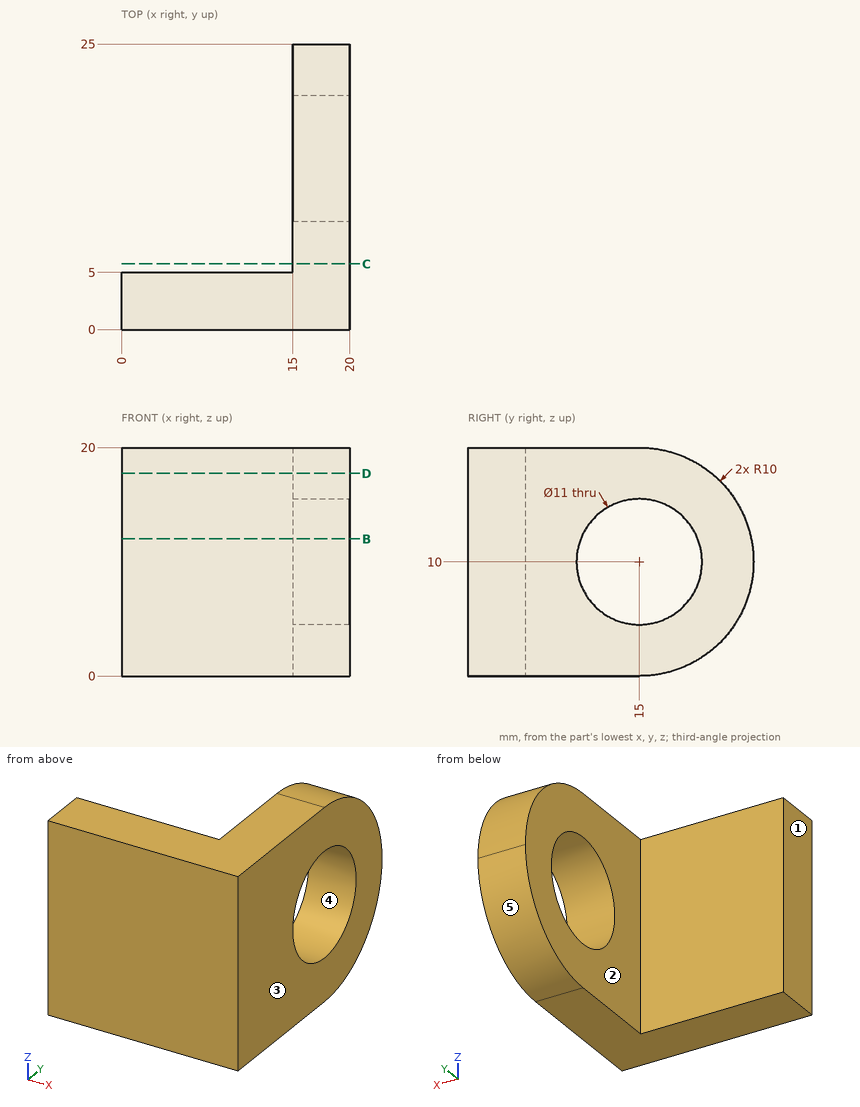
Geometry: see drawing. Coordinates: mm, zero at the bounding-box minimum. A direction names the side the tool comes from. Coordinates: 2 decimals unless noted, no trailing zeros. Order: outer loops, then holes, each group sorted by start corner. A loop starts at its lowest first (then second) coordinate and runs counter-clockwise, first axis right, second up. Notation, with made-up numbers: (89, 47.5) - (130, 47.5) arc R10 ccw to (130, 53.5) - close; hole circle Ø2 at (30.25, 41.25). An arc over 180 degrees is marked (long way). Return JSON: item names as keys, results as strings.
Q1. Access query for the marked faces 1 and 2. Directions: +Z, -Z, +X, -X, +Y, -Y. A direction counts if a zero-diameter tool reaches every point of the face in a straight line with its end or side. Return the directions, or none.
The answers:
{"face 1": "+Z, -Z, -X, +Y, -Y", "face 2": "+Z, -Z, -X, +Y"}
Q2. Cut plane C-C (y = 5.75). Return loops of the section in (x, z), then the cut area to 3 significant figures.
The answers:
{"outline": "(15, 0) - (20, 0) - (20, 20) - (15, 20) - close", "area": "100 mm2"}
Q3. Cut plane B-B (z = 12). Return loops of the section in (x, y), then the cut area to 3 significant figures.
The answers:
{"outline": "(0, 0) - (20, 0) - (20, 9.88) - (15, 9.88) - (15, 5) - (0, 5) - close; (15, 20.12) - (20, 20.12) - (20, 24.8) - (15, 24.8) - close", "area": "148 mm2"}
Q4. Draft query along Z for the marked faces 3, 4 and 5. Return one class per face: +Z half, -Z half, draft (parallel to the pull), parting line (faces both ways), or undercut.
The answers:
{"face 3": "draft", "face 4": "undercut", "face 5": "-Z half"}
Q5. Ray query, probe 1 along Y at (x, z) = (16.9, 10); probe 2 along X at (y, z) = (21.5, 8); probe 3 along Y at (x, z) = (2.5, 2.75). Return the intervals inside material, ascending.
The answers:
{"probe 1": "y = 0 to 9.5, 20.5 to 25", "probe 2": "x = 15 to 20", "probe 3": "y = 0 to 5"}
Q6. Cut plane D-D (z = 17.75). Return loops of the section in (x, y), then the cut area to 3 significant figures.
The answers:
{"outline": "(0, 0) - (20, 0) - (20, 21.32) - (15, 21.32) - (15, 5) - (0, 5) - close", "area": "182 mm2"}
Q7. First-contact query: pin 1 (1 mm diameter, centred on y = 7.5, z = 17.5, fed in from -X); pin 2 (3 mm diameter, centred on x = 17, z = 2.5, fed in from +Y); pin 3 (7.5 mm diameter, centred on x = 11, z = 10, fed in from +Y). Flat tips, straight axial feed; report the tip coordinate or a pass-through.
The answers:
{"pin 1": "stops at x = 15", "pin 2": "stops at y = 23", "pin 3": "stops at y = 5"}
